Can you work these out from the model? Positions are in its coordinate system, mm. A direction names the side the tool comes from. Round coordinates to 2 decimals unless told otherwise and drop trailing zeros. Loops run counter-clockwise (first coordinate to the right, second up) from the corner with the lowest first, then second, coordinate; pieces in that order, holes last. Notation, with made-up numbers: (64, -22) - (88, -22) arc R31 ccw to (88, 16) - close; hole circle Ø10 at (55.5, 28.25). An arc over 180 degrees is marked (long way). Answer as CSV lines item,"result".
Autodesk Inventor part; units mm, degrees
ref_plane "YZ Plane" through (0, 0, 0) normal (1, 0, 0) x (0, 1, 0)
ref_plane "XZ Plane" through (0, 0, 0) normal (0, 1, 0) x (-1, 0, 0)
ref_plane "XY Plane" through (0, 0, 0) normal (0, 0, 1) x (1, 0, 0)
sketch "Sketch1" plane through (0, 0, 0) normal (0, 0, 1) x (1, 0, 0)
  line L0 (0, 0) -> (155, 0)
  line L1 (155, 0) -> (155, 200)
  line L2 (155, 200) -> (0, 200)
  line L3 (0, 200) -> (0, 0)
  dimension "d0" = 200
  dimension "d1" = 155
extrude "Extrusion1" add sketch "Sketch1" along normal blind 5
sketch "Sketch2" plane through (0, 0, 5) normal (0, 0, 1) x (1, 0, 0)
  line L0 (155, 0) -> (155, 200)
  line L1 (155, 200) -> (0, 200)
  line L2 (0, 200) -> (0, 0)
  line L3 (0, 0) -> (155, 0)
  line L4 (2.5, 197.5) -> (152.5, 197.5)
  line L5 (152.5, 197.5) -> (152.5, 2.5)
  line L6 (152.5, 2.5) -> (2.5, 2.5)
  line L7 (2.5, 2.5) -> (2.5, 197.5)
  dimension "d4" = 150
  dimension "d5" = 195
  dimension "d6" = 2.5
  dimension "d7" = 2.5
extrude "Extrusion2" cut sketch "Sketch2" against normal up to surface (5 mm away) contours L4 L5 L6 L7
properties part number "rubberSeal"
Q1. Imagine slicing it at A-A (x = 122). Write out the boundary of the cut face in (y, z).
Checks:
outline,"(0, 0) - (2.5, 0) - (2.5, 5) - (0, 5) - close; (197.5, 0) - (200, 0) - (200, 5) - (197.5, 5) - close"
Q2. On a 3-axis mill with a long thin cutter (end or side, diameter ignored), from which of +Z, -Z, +X, -X, +Y, -Y can I reach the whole of each face in a straight line? I mean faces 4 (the flat face through (79, 2.5, 3)), 5 (the flat face through (155, 99, 2)). Say none if no direction works.
Checks:
face 4,"+Z, -Z"
face 5,"+Z, -Z, +X, +Y, -Y"
Q3. We'd pull the mould along X, two halves only. Please class faces 1 (the flat face through (0, 101, 2)), 2 (the flat face through (76, 197.5, 3)), 3 (the flat face through (79, 200, 2)): pulls with the +X half, pulls with the -X half, needs draft (parallel to the pull), parting line crosses it, or undercut.
Checks:
face 1,"pulls with the -X half"
face 2,"undercut"
face 3,"needs draft"
Q4. Imagine slicing it at C-C (z = 3.35). Write out the boundary of the cut face in (x, y), then the cut area to 3 significant figures.
Checks:
outline,"(0, 0) - (155, 0) - (155, 200) - (0, 200) - close; hole (2.5, 2.5) - (152.5, 2.5) - (152.5, 197.5) - (2.5, 197.5) - close"
area,"1,750 mm²"
Q5. Imagine slicing it at B-B (y = 133). Write out the boundary of the cut face in (x, z), then the cut area to 3 significant figures.
Checks:
outline,"(0, 0) - (2.5, 0) - (2.5, 5) - (0, 5) - close; (152.5, 0) - (155, 0) - (155, 5) - (152.5, 5) - close"
area,"25.0 mm²"
Q6. If I drill on line 1 along X through (y, z) = (176, 2.05); line 2 along Y through (x, z) = (126.5, 3.3), over which ranges is the centre line in solid material (lowest first)? Write a range as [from, to].
Checks:
line 1,"[0, 2.5], [152.5, 155]"
line 2,"[0, 2.5], [197.5, 200]"
